For this review, take the finished solid that the model builds, in its own axes (mm). Give positions to 0.01 mm unless a question says otherwise; leave off trailing zeros. Loops run counter-clockwise (first coordinate to the right, second up) from the corner with the lowest first, then second, coordinate; pieces in that order, holes last. Notation, with made-up numbers: (56, 53.25) - (78, 53.25) arc R22 cw to (78, 65.25) - close; hole circle Ø2 at (-15, 35). An arc over 180 degrees is marked (long way). Use CSV: the item, a comma, the result in double quotes. Start each with the question number.
1. Take a section at B-B on x = 76.5. Give the boundary of the cut face in (y, z), plus the area to 3 significant figures.
2. Wall thickness on line 1 (Y direction, x = 187.6, z = 1.15); line 2 (Y direction, x = 120, z = 0.5); line 3 (X direction, y = 9.5, z = 0.3): over which ranges is each line inside the solid? List them lowest first.
3. Take a section at A-A on z = 1.3. State how many separate pieces and enclosed holes the cut face has, plus the area to 3 significant figures.
4. For pin 1 (1 mm diameter, centred on y = -52, z = 1.5, fed in from +X); pin 2 (1 mm diameter, centred on x = 37, z = 1, fed in from -Y); pin 3 (0.6 mm diameter, centred on x = -186, z = 1, fed in from +Y), all flat-tipped, find the tip position at first contact; note any pin that passes through.
5. Take a section at C-C on y = 49.5. Give the boundary of the cut face in (x, z), plus the area to 3 significant figures.
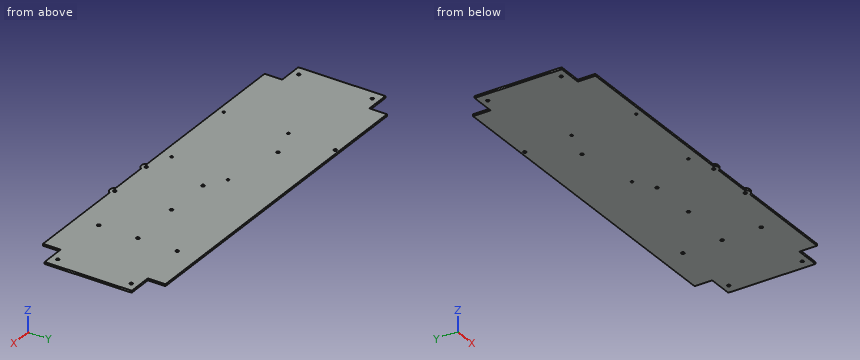
```python
from build123d import *

# Parameters (mm, degrees)
SKETCH1_W               = 395
SKETCH1_H               = 125
BOSS_EXTRUDE1_DEPTH     = 2
SKETCH2_R               = 1.55
FIXING_HOLES_DEPTH      = 208.162979318
SKETCH3_W               = 25
SKETCH3_H               = 18
CUT_EXTRUDE2_DEPTH      = 208.162979318
MIRROR2_COPY_1_SKETCH_W = 25
MIRROR2_COPY_1_SKETCH_H = 18
MIRROR2_COPY_1_DEPTH    = 208.162979318
SKETCH4_R               = 1.25
CAVE_BOARD_HOLES_DEPTH  = 208.162979318
SKETCH5_R               = 1.6
RPI_HOLES_DEPTH         = 208.162979318
SKETCH6_R               = 1.6
BUZZER_HOLES_DEPTH      = 208.162979318
SKETCH7_R               = 1.6
RELAYS_HOLES_DEPTH      = 208.162979318
BOSS_EXTRUDE2_DEPTH     = 2


with BuildPart() as part:
    # Sketch1 → Boss-Extrude1 (new body)
    with BuildSketch(Plane.XY):
        Rectangle(SKETCH1_W, SKETCH1_H)
    extrude(amount=BOSS_EXTRUDE1_DEPTH)

    # Sketch2 → Fixing_holes (cut, through all)
    with BuildSketch(Plane.XY.offset(2)):
        with Locations((-187.6, 37.5)):
            Circle(SKETCH2_R)
        with Locations((-187.6, -37.5)):
            Circle(SKETCH2_R)
        with Locations((187.6, 37.5)):
            Circle(SKETCH2_R)
        with Locations((187.6, -37.5)):
            Circle(SKETCH2_R)
    extrude(amount=-FIXING_HOLES_DEPTH, mode=Mode.SUBTRACT)

    # Sketch3 → Cut-Extrude2 (cut, through all)
    with BuildSketch(Plane.XY.offset(2)):
        with Locations((-185, 53.5)):
            Rectangle(SKETCH3_W, SKETCH3_H)
    cut_extrude2 = extrude(amount=-CUT_EXTRUDE2_DEPTH, mode=Mode.SUBTRACT)

    # Mirror1: Cut-Extrude2 across plane
    add(cut_extrude2.mirror(Plane.ZX), mode=Mode.SUBTRACT)

    # Mirror2: Cut-Extrude2 across plane
    add(cut_extrude2.mirror(Plane(origin=(0, 0, 0), x_dir=(0, 0, 1), z_dir=(1, 0, 0))), mode=Mode.SUBTRACT)

    # Mirror2 copy 1 sketch → Mirror2 copy 1 (cut, through all)
    with BuildSketch(Plane(origin=(0, 0, 2), x_dir=(-1, 0, 0), z_dir=(0, 0, 1))):
        with Locations((-185, 53.5)):
            Rectangle(MIRROR2_COPY_1_SKETCH_W, MIRROR2_COPY_1_SKETCH_H)
    extrude(amount=-MIRROR2_COPY_1_DEPTH, mode=Mode.SUBTRACT)

    # Sketch4 → Cave_board_holes (cut, through all)
    with BuildSketch(Plane.XY.offset(2)):
        with Locations((-99, 10)):
            Circle(SKETCH4_R)
        with Locations((-99, -56)):
            Circle(SKETCH4_R)
        with Locations((-5, 10)):
            Circle(SKETCH4_R)
        with Locations((-11, -51.5)):
            Circle(SKETCH4_R)
    extrude(amount=-CAVE_BOARD_HOLES_DEPTH, mode=Mode.SUBTRACT)

    # Sketch5 → RPi_holes (cut, through all)
    with BuildSketch(Plane.XY.offset(2)):
        with Locations((15, -2.4)):
            Circle(SKETCH5_R)
        with Locations((15, -60.4)):
            Circle(SKETCH5_R)
        with Locations((64, -2.4)):
            Circle(SKETCH5_R)
        with Locations((64, -60.4)):
            Circle(SKETCH5_R)
    extrude(amount=-RPI_HOLES_DEPTH, mode=Mode.SUBTRACT)

    # Sketch6 → buzzer_holes (cut, through all)
    with BuildSketch(Plane.XY.offset(2)):
        with Locations((-97.5, 59)):
            Circle(SKETCH6_R)
        with Locations((-67.5, 20)):
            Circle(SKETCH6_R)
    extrude(amount=-BUZZER_HOLES_DEPTH, mode=Mode.SUBTRACT)

    # Sketch7 → relays_holes (cut, through all)
    with BuildSketch(Plane.XY.offset(2)):
        with Locations((120, 0)):
            Circle(SKETCH7_R)
        with Locations((120, 40)):
            Circle(SKETCH7_R)
        with Locations((120, -40)):
            Circle(SKETCH7_R)
    extrude(amount=-RELAYS_HOLES_DEPTH, mode=Mode.SUBTRACT)

    # Sketch8 → Boss-Extrude2 (add)
    with BuildSketch(Plane.XY.offset(2)):
        with BuildLine():
            Line((10.462379478, -62.5), (19.537620522, -62.5))
            ThreePointArc((19.537620522, -62.5), (15, -65.4), (10.462379478, -62.5))
        make_face()
        with BuildLine():
            Line((59.462379478, -62.5), (68.537620522, -62.5))
            ThreePointArc((68.537620522, -62.5), (64, -65.4), (59.462379478, -62.5))
        make_face()
    extrude(amount=-BOSS_EXTRUDE2_DEPTH)


solid = part.part
```
Check result:
1,outline,"(-62.5, 0) - (62.5, 0) - (62.5, 2) - (-62.5, 2) - close"
1,area,"250 mm²"
2,line 1,"y = -44.5 to -39.05, -35.95 to 35.95, 39.05 to 44.5"
2,line 2,"y = -62.5 to -41.6, -38.4 to -1.6, 1.6 to 38.4, 41.6 to 62.5"
2,line 3,"x = -197.5 to -100.15, -97.85 to -6.15, -3.85 to 197.5"
3,separate pieces,"1"
3,enclosed holes,"17"
3,area,"47,500 mm²"
4,pin 1,"stops at x = 172.5"
4,pin 2,"stops at y = -62.5"
4,pin 3,"stops at y = 44.5"
5,outline,"(-172.5, 0) - (172.5, 0) - (172.5, 2) - (-172.5, 2) - close"
5,area,"690 mm²"
